from build123d import *

# Parameters (mm, degrees)
BOSS_EXTRUDE1_DEPTH = 10
SKETCH2_W           = 23
SKETCH2_H           = 23
BOSS_EXTRUDE2_DEPTH = 1


with BuildPart() as part:
    # Sketch1 → Boss-Extrude1 (new body)
    with BuildSketch(Plane(origin=(0, 0, 0), x_dir=(1, 0, 0), z_dir=(0, 1, 0))):
        Polygon((-36.489872914, 17.750117647), (-36.489872914, -2.249882353), (-13.489872914, -2.249882353), (-13.489872914, 0.750117647), (-33.489872914, 0.750117647), (-33.489872914, 20.750117647), (-36.489872914, 20.750117647), align=None)
    extrude(amount=BOSS_EXTRUDE1_DEPTH)

    # Sketch2 → Boss-Extrude2 (add)
    with BuildSketch(Plane.XZ):
        with Locations((-24.989872914, -9.250117647)):
            Rectangle(SKETCH2_W, SKETCH2_H)
    extrude(amount=BOSS_EXTRUDE2_DEPTH)


solid = part.part
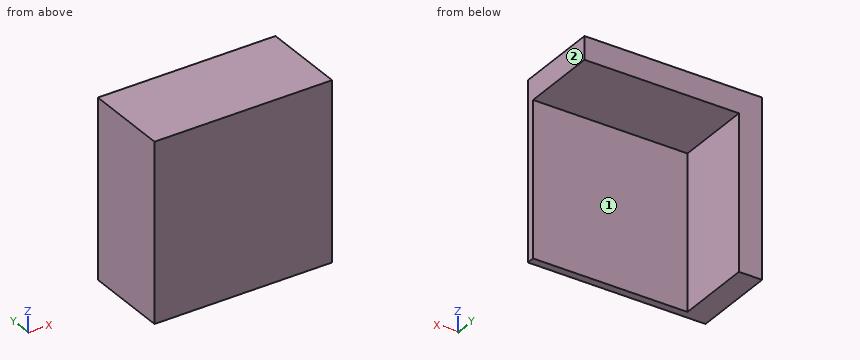
Input: part model. Units: mm. Frame: model coordinates. Face numbers are marked on the shaded views. A direction names the side the tool comes from. Give positions to 0.01 mm unless a question says otherwise; leave off trailing zeros. Loops run counter-clockwise (first coordinate to the right, second up) from the corner with the lowest first, then second, coordinate; pieces in that order, holes last. Notation, with made-up numbers: M 19,-24.5 L 39,-24.5 A15 cw 39,-8.5 Z; hole C 31,-16 d5. An arc over 180 degrees is marked long. Use CSV: the item, a comma, the result in double quotes.
(1) Set-up query: the marked faces 1 and 2. Return all of +Z, -Z, +X, -X, +Y, -Y with unobstructed straight access to the full face (end or side cutting, diameter ignored); none if empty.
Outcome:
face 1,"-Z, +X, +Y"
face 2,"+Z, -Z, +X, +Y, -Y"
(2) Pin query (flat end, axial travel): P1, Ø1.5, axis at x = -29.5, z = -9.5, coming from the +Y side; P2, Ø3, axis at y = 8, z = -5, coming from the +X side. Return the tip coordinate at first contact, or that it passes through.
Outcome:
P1,"stops at y = 0"
P2,"stops at x = -33.49"
(3) Section A-A, the plane z = -16.5. Return loops of the section in (x, y), plus the area to 3 significant figures.
Outcome:
outline,"M -36.49,-1 L -13.49,-1 L -13.49,0 L -33.49,0 L -33.49,10 L -36.49,10 Z"
area,"53.0 mm²"
(4) Section B-B, the plane x = -31.5. Return loops of the section in (y, z).
Outcome:
outline,"M -1,-20.75 L 0,-20.75 L 0,-0.75 L 10,-0.75 L 10,2.25 L -1,2.25 Z"
(5) Material intervals for L1, parallel to Y at x = -27, z = -4.5; L2, parallel to Z at x = -24.75, y = 2.75; L3, parallel to X at y = 2.75, z = -8.75, sorted ascending. Write a range as [from, to].
Outcome:
L1,"y = [-1, 0]"
L2,"z = [-0.75, 2.25]"
L3,"x = [-36.49, -33.49]"
